Check sheet for the drawn part. Datum: minimum x, y, z corner. Units: mm. Coordinates: 2 decimals unless noted, no trailing zeros. Order: outer loops, then holes, each group sorted by start corner. A loop starts at its lowest first (then second) coordinate and runs counter-clockwise, first axis right, second up. Notation, with made-up numbers: M 62,-5 L 81,-5 A25 cw 81,14 Z; hole C 42.5,31 d7. An arc over 180 degrees is marked long. Answer in a Markdown table with one row per item. Add a question column.
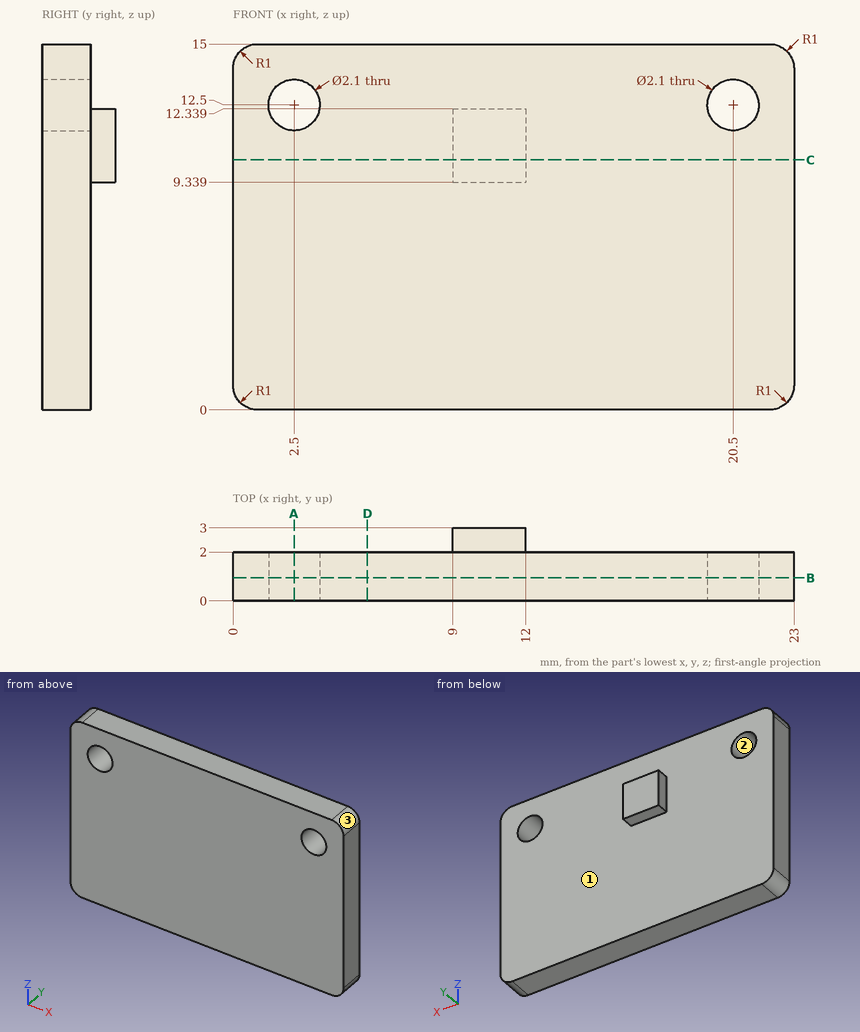
1. Go/stop test with flat-tipped pins: pin 1 Ø0.8 at (x, y) = (11, 2.5) entering from +Z; pin 2 Ø6 at (x, z) = (4.5, 5) entering from +Y; pin 3 Ø1.9 at (x, z) = (20.5, 12.5) entering from -Y. Record where each tip stops, or that it passes through.
2. Section check B-B on y = 0.95. Enter the section's corners in (x, z).
3. Release check for a two-part mould opening along X. For the marked faces 1, 2 and 3 record: released by +X, released by -X, zero draft, split by the parting line, or undercut.
4. Scan lines: line 1 (X direction, y = 1.35, z = 12.5); line 2 (Z direction, x = 20.5, y = 0.7); line 3 (Y direction, x = 4, z = 12.5). Record each from-to range of solid material in increasing order.
5. Section check D-D on x = 5.5. Enter the section's corners in (y, z).
6. Section check C-C on z = 10.25. Enter the section's corners in (x, y).
7. Section check A-A on x = 2.5. Enter the section's corners in (y, z).
Result sheet:
| question | item | result |
|---|---|---|
| 1 | pin 1 | z = 12.34 |
| 1 | pin 2 | y = 2 |
| 1 | pin 3 | through |
| 2 | outline | M 0,1 A1 ccw 1,0 L 22,0 A1 ccw 23,1 L 23,14 A1 ccw 22,15 L 1,15 A1 ccw 0,14 Z; hole C 2.5,12.5 d2.1; hole C 20.5,12.5 d2.1 |
| 3 | face 1 | zero draft |
| 3 | face 2 | undercut |
| 3 | face 3 | released by +X |
| 4 | line 1 | 0 to 1.45, 3.55 to 19.45, 21.55 to 23 |
| 4 | line 2 | 0 to 11.45, 13.55 to 15 |
| 4 | line 3 | 0 to 2 |
| 5 | outline | M 0,0 L 2,0 L 2,15 L 0,15 Z |
| 6 | outline | M 0,0 L 23,0 L 23,2 L 12,2 L 12,3 L 9,3 L 9,2 L 0,2 Z |
| 7 | outline | M 0,0 L 2,0 L 2,11.45 L 0,11.45 Z; M 0,13.55 L 2,13.55 L 2,15 L 0,15 Z |
